Here's how the part is built. I have some questions about the finished solid (model axes, mm). A direction names the side the tool comes from. Give positions to 0.01 mm unless a question says otherwise; leave off trailing zeros. Loops run counter-clockwise (first coordinate to the right, second up) from the corner with the lowest first, then second, coordinate; pieces in that order, holes last. Notation, with made-up numbers: (-36, 43.5) - (-19, 43.5) arc R16 cw to (-19, 57.5) - close; hole circle Ø1 at (-5.75, -14.75). An arc over 180 degrees is marked (long way). Put each result on its own line as item: value. Start each with the question number.
from build123d import *

# Parameters (mm, degrees)
F1_DEPTH       = 35
F3_D           = 5
F3_START       = 1.7550021
F3_CBORE_D     = 10
F3_CBORE_DEPTH = 8
F4_W           = 22.4
F4_H           = 2
F5_DEPTH       = 25
F6_R           = 6
F7_DEPTH       = 8


with BuildPart() as f1:
    # F0 (on Top) → F1 (new body, symmetric)
    with BuildSketch(Plane.XY):
        with BuildLine():
            ThreePointArc((-17.3192642082, 2.5086026559), (17.5, 0), (-17.3192642082, -2.5086026559))
            Line((-17.3192642082, -2.5086026559), (-20.3459311096, -2.5086026559))
            ThreePointArc((-20.3459311096, -2.5086026559), (-16.3392263155, -12.3806172468), (-7.9192642082, -18.9086026559))
            ThreePointArc((-7.9192642082, -18.9086026559), (20.5, 0), (-7.9192642082, 18.9086026559))
            Line((-7.9192642082, 18.9086026559), (-20.1192642082, 18.9086026559))
            ThreePointArc((-20.1192642082, 18.9086026559), (-25.7761184577, 16.5654569054), (-28.1192642082, 10.9086026559))
            Line((-28.1192642082, 10.9086026559), (-28.1192642082, 2.5086026559))
            Line((-28.1192642082, 2.5086026559), (-17.3192642082, 2.5086026559))
        make_face()
        with BuildLine():
            ThreePointArc((-7.9192642082, -18.9086026559), (-16.3392263155, -12.3806172468), (-20.3459311096, -2.5086026559))
            Line((-20.3459311096, -2.5086026559), (-28.1192642082, -2.5086026559))
            Line((-28.1192642082, -2.5086026559), (-28.1192642082, -10.9086026559))
            ThreePointArc((-28.1192642082, -10.9086026559), (-25.7761184577, -16.5654569054), (-20.1192642082, -18.9086026559))
            Line((-20.1192642082, -18.9086026559), (-7.9192642082, -18.9086026559))
        make_face()
    extrude(amount=F1_DEPTH, both=True)

    # F3 (through all)
    # its depths count from where the whole tool has entered the part; down to there all is cleared
    with Locations(Plane.XZ.offset(18.9086026559).offset(-F3_START)):
        with Locations((-20.1192642082, -24.25), (-20.1192642082, -9.25), (-20.1192642082, 9.25), (-20.1192642082, 24.25)):
            CounterBoreHole(F3_D / 2, F3_CBORE_D / 2, F3_CBORE_DEPTH)

    # F4 (on Front) → F5 (cut, symmetric)
    with BuildSketch(Plane.XZ):
        with Locations((-16.8941898715, -1)):
            Rectangle(F4_W, F4_H)
    extrude(amount=F5_DEPTH, both=True, mode=Mode.SUBTRACT)

    # F6 (on Top) → F7 (cut)
    with BuildSketch(Plane.XY):
        with Locations((0, -25)):
            Circle(F6_R)
        with Locations((17.6776695297, -17.6776695297)):
            Circle(F6_R)
        with Locations((25, 0)):
            Circle(F6_R)
        with Locations((17.6776695297, 17.6776695297)):
            Circle(F6_R)
        with Locations((0, 25)):
            Circle(F6_R)
    extrude(amount=-F7_DEPTH, mode=Mode.SUBTRACT)


solid = f1.part
1) Suppose I cut it at A-A on x = 0. Please give me the cut outline in (y, z).
2) Suppose I cut it at B-B on z = 30.5. Please give me the cut outline in (x, y).
3) Suppose I cut it at D-D on z = 9.25. Please give me the cut outline in (x, y).
4) Which directions (+Z, -Z, +X, -X, +Y, -Y) give clear straight access to the entire face, cutting with the end or side of a thin tool? Please do faces 4 (the cylindrical face through (13.47, -13.4, -3.94)), 5 (the cylindrical face through (0, -19, -4)), 6 (the flat face through (14, 14, 0)).
5) I need wall thicknesses on line 1 (X direction, y = -6, z = 24); line 2 (X direction, y = 12, z = 8.5); line 3 (X direction, y = 7, z = 32.5). Which ranges of each line are inside material? Lowest first, please.
6) I'm going to push flat-ended pins straight in: P1, Ø5, axis at x = -8, z = -18.5, coming from the -Y side; P2, Ø3, axis at x = -20.12, z = 9.25, coming from the +Y side; P3, Ø16, axis at x = -20.12, z = 24.25, coming from the -Y side; P4, Ø12, axis at x = -12, z = 11.5, coming from the -Y side. Where does each tip first touch, or does it pass through?
7) Suppose I cut it at C-C on y = -8. Please give me the cut outline in (x, z).
8) Thinking about a two-plate mould opening in X: for faces 1 (the cylindrical face through (19, 0, -4)), 2 (the cylindrical face through (-22.429, 10.823, 8.292)), 3 (the flat face through (-22.8, 2.509, 0.5)), which applies, pulls with the +X half, pulls with the -X half, needs draft (parallel to the pull), parting line crosses it, or undercut?
Ans:
1. outline: (-20.5, -35) - (-17.5, -35) - (-17.5, 35) - (-20.5, 35) - (-20.5, 0) - (-19, 0) - (-19, -8) - (-20.5, -8) - close; (17.5, -35) - (20.5, -35) - (20.5, -8) - (19, -8) - (19, 0) - (20.5, 0) - (20.5, 35) - (17.5, 35) - close
2. outline: (-28.12, -10.91) arc R8 ccw to (-20.12, -18.91) - (-7.92, -18.91) arc R20.5 ccw (long way) to (-7.92, 18.91) - (-20.12, 18.91) arc R8 ccw to (-28.12, 10.91) - (-28.12, 2.51) - (-17.32, 2.51) arc R17.5 cw (long way) to (-17.32, -2.51) - (-28.12, -2.51) - close
3. outline: (-28.12, -10.91) arc R8 ccw to (-25.12, -17.15) - (-25.12, -9.15) - (-22.62, -9.15) - (-22.62, -2.51) - (-28.12, -2.51) - close; (-28.12, 2.51) - (-22.62, 2.51) - (-22.62, 18.51) arc R8 ccw to (-28.12, 10.91) - close; (-17.62, -9.15) - (-15.12, -9.15) - (-15.12, -18.91) - (-7.92, -18.91) arc R20.5 ccw (long way) to (-7.92, 18.91) - (-17.62, 18.91) - (-17.62, 2.51) - (-17.32, 2.51) arc R17.5 cw (long way) to (-17.32, -2.51) - (-17.62, -2.51) - close
4. face 4: +X, -Y
4. face 5: -Y
4. face 6: +X, +Y
5. line 1: x = -28.12 to -22.61, -17.63 to -16.44, 16.44 to 19.6
5. line 2: x = -28.04 to -22.5, -17.73 to -12.74, 12.74 to 16.62
5. line 3: x = -28.12 to -16.04, 16.04 to 19.27
6. P1: stops at y = -19.75
6. P2: passes through
6. P3: stops at y = -18.91
6. P4: stops at y = -19.6
7. outline: (-28.12, -35) - (-15.56, -35) - (-15.56, -2) - (-28.09, -2) - (-28.09, 0) - (-15.56, 0) - (-15.56, 35) - (-28.12, 35) - close; (15.56, -35) - (18.87, -35) - (18.87, 35) - (15.56, 35) - close; hole circle Ø5 at (-20.12, -24.25); hole circle Ø5 at (-20.12, -9.25); hole circle Ø5 at (-20.12, 9.25); hole circle Ø5 at (-20.12, 24.25)
8. face 1: pulls with the +X half
8. face 2: undercut
8. face 3: needs draft
